from build123d import *

# Parameters (mm, degrees)
SKETCH_1_R               = 2.1
SKETCH_1_W               = 60
SKETCH_1_H               = 60
SKETCH_1_W_2             = 55
SKETCH_1_H_2             = 55
EXTRUDE_1_DEPTH          = 15
CUT_EXTRUDE_1_DEPTH      = 160.024864418
CUT_EXTRUDE_1_DEPTH_BACK = 160.024864418
CUT_EXTRUDE_2_DEPTH      = 184.645620758
CUT_EXTRUDE_2_DEPTH_BACK = 184.645620758


with BuildPart() as part:
    # Эскиз1 → Бобышка-Вытянуть1 (new body)
    # profile 1 of 13: a face of its own
    with BuildSketch(Plane(origin=(0, 45.645974268, 0), x_dir=(-1, 0, 0), z_dir=(0, -1, 0))):
        Polygon((-109.808980694, -130.773129836), (-128.058980694, -130.773129836), (-128.058980694, -48.273129836), (-109.808980694, -48.273129836), (-109.808980694, -53.898129836), (-124.808980694, -53.898129836), (-124.808980694, -125.148129836), (-109.808980694, -125.148129836), align=None)
    # profile 2 of 13: a face of its own
    with BuildSketch(Plane(origin=(0, 45.645974268, 0), x_dir=(-1, 0, 0), z_dir=(0, -1, 0))):
        Polygon((-109.808980694, -130.773129836), (-99.808980694, -130.773129836), (-99.808980694, -124.523129836), (-99.808980694, -119.523129836), (-99.808980694, -95.523129836), (-99.808980694, -83.523129836), (-99.808980694, -59.523129836), (-99.808980694, -54.523129836), (-99.808980694, -48.273129836), (-109.808980694, -48.273129836), (-109.808980694, -53.898129836), (-109.808980694, -125.148129836), align=None)
        with Locations(Location((-104.808980694, -119.523129836, 0), (0, 0, 90))):
            Circle(SKETCH_1_R, mode=Mode.SUBTRACT)
        with Locations(Location((-104.808980694, -59.523129836, 0), (0, 0, 90))):
            Circle(SKETCH_1_R, mode=Mode.SUBTRACT)
    # profile 3 of 13: a face of its own
    with BuildSketch(Plane(origin=(0, 45.645974268, 0), x_dir=(-1, 0, 0), z_dir=(0, -1, 0))):
        with Locations((-64.808980694, -89.523129836)):
            Rectangle(SKETCH_1_W, SKETCH_1_H)
        with Locations((-64.5, -89.5)):
            Rectangle(SKETCH_1_W_2, SKETCH_1_H_2, mode=Mode.SUBTRACT)
    # profile 4 of 13: a face of its own
    with BuildSketch(Plane(origin=(0, 45.645974268, 0), x_dir=(-1, 0, 0), z_dir=(0, -1, 0))):
        Polygon((-64.808980694, -124.523129836), (-55, -124.523129836), (-55, -119.523129836), (-75, -119.523129836), (-75, -124.523129836), align=None)
    # profile 5 of 13: a face of its own
    with BuildSketch(Plane(origin=(0, 45.645974268, 0), x_dir=(-1, 0, 0), z_dir=(0, -1, 0))):
        Polygon((-99.808980694, -130.773129836), (-99.808980694, -124.523129836), (-64.808980694, -124.523129836), (-29.808980694, -124.523129836), (-29.808980694, -130.773129836), align=None)
    # profile 6 of 13: a face of its own
    with BuildSketch(Plane(origin=(0, 45.645974268, 0), x_dir=(-1, 0, 0), z_dir=(0, -1, 0))):
        Polygon((-99.808980694, -54.523129836), (-99.808980694, -48.273129836), (-29.808980694, -48.273129836), (-29.808980694, -54.523129836), (-64.808980694, -54.523129836), align=None)
    # profile 7 of 13: a face of its own
    with BuildSketch(Plane(origin=(0, 45.645974268, 0), x_dir=(-1, 0, 0), z_dir=(0, -1, 0))):
        Polygon((-29.808980694, -130.773129836), (-29.808980694, -124.523129836), (-29.808980694, -54.523129836), (-29.808980694, -48.273129836), (-19.808980694, -48.273129836), (-19.808980694, -53.898129836), (-19.808980694, -125.148129836), (-19.808980694, -130.773129836), align=None)
        with Locations(Location((-24.808980694, -119.523129836, 0), (0, 0, 90))):
            Circle(SKETCH_1_R, mode=Mode.SUBTRACT)
        with Locations(Location((-24.808980694, -59.523129836, 0), (0, 0, 90))):
            Circle(SKETCH_1_R, mode=Mode.SUBTRACT)
    # profile 8 of 13: a face of its own
    with BuildSketch(Plane(origin=(0, 45.645974268, 0), x_dir=(-1, 0, 0), z_dir=(0, -1, 0))):
        Polygon((-4.808980694, -125.148129836), (-4.808980694, -53.898129836), (-19.808980694, -53.898129836), (-19.808980694, -48.273129836), (-1.558980694, -48.273129836), (-1.558980694, -130.773129836), (-19.808980694, -130.773129836), (-19.808980694, -125.148129836), align=None)
    # profile 9 of 13: a face of its own
    with BuildSketch(Plane(origin=(0, 45.645974268, 0), x_dir=(-1, 0, 0), z_dir=(0, -1, 0))):
        Polygon((-99.808980694, -119.523129836), (-99.808980694, -124.523129836), (-94.808980694, -124.523129836), (-89.808980694, -119.523129836), (-94.808980694, -119.523129836), (-94.808980694, -114.523129836), align=None)
    # profile 10 of 13: a face of its own
    with BuildSketch(Plane(origin=(0, 45.645974268, 0), x_dir=(-1, 0, 0), z_dir=(0, -1, 0))):
        Polygon((-34.808980694, -124.523129836), (-29.808980694, -124.523129836), (-29.808980694, -119.523129836), (-34.808980694, -114.523129836), (-34.808980694, -119.523129836), (-39.808980694, -119.523129836), align=None)
    # profile 11 of 13: a face of its own
    with BuildSketch(Plane(origin=(0, 45.645974268, 0), x_dir=(-1, 0, 0), z_dir=(0, -1, 0))):
        Polygon((-34.808980694, -64.523129836), (-29.808980694, -59.523129836), (-29.808980694, -54.523129836), (-34.808980694, -54.523129836), (-39.808980694, -59.523129836), (-34.808980694, -59.523129836), align=None)
    # profile 12 of 13: a face of its own
    with BuildSketch(Plane(origin=(0, 45.645974268, 0), x_dir=(-1, 0, 0), z_dir=(0, -1, 0))):
        Polygon((-99.808980694, -54.523129836), (-99.808980694, -59.523129836), (-94.808980694, -64.523129836), (-94.808980694, -59.523129836), (-89.808980694, -59.523129836), (-94.808980694, -54.523129836), align=None)
    # profile 13 of 13: a face of its own
    with BuildSketch(Plane(origin=(0, 45.645974268, 0), x_dir=(-1, 0, 0), z_dir=(0, -1, 0))):
        Polygon((-55, -59.523129836), (-55, -54.523129836), (-64.808980694, -54.523129836), (-75, -54.523129836), (-75, -59.523129836), align=None)
    extrude(amount=EXTRUDE_1_DEPTH)

    # Эскиз2 → Вырез-Вытянуть1 (cut, two sides: drawn at the far end of the back side and taken through both)
    with BuildSketch(Plane.XY.offset(130.773129836).offset(-CUT_EXTRUDE_1_DEPTH_BACK)):
        Polygon((64.808980694, 44), (72, 44), (72, 37), (58, 37), (58, 44), align=None)
    extrude(amount=CUT_EXTRUDE_1_DEPTH + CUT_EXTRUDE_1_DEPTH_BACK, mode=Mode.SUBTRACT)

    # Эскиз3 → Вырез-Вытянуть2 (cut, two sides: drawn at the far end of the back side and taken through both)
    with BuildSketch(Plane(origin=(0, 45.645974268, 0), x_dir=(1, 0, 0), z_dir=(0, 1, 0)).offset(-CUT_EXTRUDE_2_DEPTH_BACK)):
        Polygon((103.808980694, -70.898129836), (103.808980694, -109.148129836), (109.808980694, -115.148129836), (109.808980694, -63.898129836), align=None)
        Polygon((25.808980694, -70.898129836), (25.808980694, -109.148129836), (19.808980694, -115.148129836), (19.808980694, -63.898129836), align=None)
    extrude(amount=CUT_EXTRUDE_2_DEPTH + CUT_EXTRUDE_2_DEPTH_BACK, mode=Mode.SUBTRACT)


solid = part.part
Geometry: final body of the model. Coordinates: model frame, mm. A direction names the side the tool comes from. Round coordinates to 2 decimals unless told otherwise and drop trailing zeros. Order: outer loops, then holes, each group sorted by start corner. A loop starts at its lowest first (then second) coordinate and runs counter-clockwise, first axis right, second up.
Q1. Section B-B, the plane z = 77. Output: boundary loops of the cut face in (x, y), and give its area (4 significant figures).
Result sheet:
outline: (1.56, 30.65) - (4.81, 30.65) - (4.81, 45.65) - (1.56, 45.65) - close; (25.81, 30.65) - (29.81, 30.65) - (29.81, 45.65) - (25.81, 45.65) - close; (34.81, 30.65) - (37, 30.65) - (37, 45.65) - (34.81, 45.65) - close; (92, 30.65) - (94.81, 30.65) - (94.81, 45.65) - (92, 45.65) - close; (99.81, 30.65) - (103.81, 30.65) - (103.81, 45.65) - (99.81, 45.65) - close; (124.81, 30.65) - (128.06, 30.65) - (128.06, 45.65) - (124.81, 45.65) - close
area: 292.5 mm2
Q2. Material intervals for probe 1 along X at (y, z) = (34.5, 82); probe 2 along Z at (x, y) = (49.5, 39.75); probe 3 along Z at (x, y) = (57, 38.75), sorted ascending.
Result sheet:
probe 1: x = 1.56 to 4.81, 25.81 to 29.81, 34.81 to 37, 92 to 94.81, 99.81 to 103.81, 124.81 to 128.06
probe 2: z = 48.27 to 54.52, 59.52 to 62, 117 to 119.52, 124.52 to 130.77
probe 3: z = 48.27 to 62, 117 to 130.77
Q3. Access query for faces 1 (the face through (65, 37, 124)), 2 (the face through (1.559, 38, 89)), 3 (the face through (109.809, 38, 120)). Directions: +Z, -Z, +X, -X, +Y, -Y. A direction counts if a zero-diameter tool reaches every point of the face in a straight line with its end or side. Return the directions, or none.
Result sheet:
face 1: +Z, -Z
face 2: +Z, -Z, -X, +Y, -Y
face 3: +Y, -Y
Q4. Mould query, pull axis Z, two halves, no side actions, for faces 4 (the face through (97.274, 38.251, 116.988)), 5 (the face through (63.9, 36.6, 130.773)), 6 (the face through (65.7, 36.6, 48.273)), 7 (the face through (128.059, 38, 90)). Classes: released by +Z, released by -Z, zero draft, split by the parting line, or undercut.
Result sheet:
face 4: undercut
face 5: released by +Z
face 6: released by -Z
face 7: zero draft
Q5. Section D-D, the plane x = 41.5. Output: boundary loops of the cut face in (y, z).
Result sheet:
outline: (30.65, 48.27) - (45.65, 48.27) - (45.65, 54.52) - (30.65, 54.52) - close; (30.65, 59.52) - (45.65, 59.52) - (45.65, 62) - (30.65, 62) - close; (30.65, 117) - (45.65, 117) - (45.65, 119.52) - (30.65, 119.52) - close; (30.65, 124.52) - (45.65, 124.52) - (45.65, 130.77) - (30.65, 130.77) - close
Q6. Section C-C, the plane x = 14. Output: boundary loops of the cut face in (y, z), and give its area (3 significant figures).
Result sheet:
outline: (30.65, 48.27) - (45.65, 48.27) - (45.65, 53.9) - (30.65, 53.9) - close; (30.65, 125.15) - (45.65, 125.15) - (45.65, 130.77) - (30.65, 130.77) - close
area: 169 mm2
Q7. Section A-A, the plane x = 70.5. Output: boundary loops of the cut face in (y, z), and give its area (3 significant figures).
Result sheet:
outline: (30.65, 48.27) - (37, 48.27) - (37, 62) - (30.65, 62) - close; (30.65, 117) - (37, 117) - (37, 130.77) - (30.65, 130.77) - close; (44, 48.27) - (45.65, 48.27) - (45.65, 62) - (44, 62) - close; (44, 117) - (45.65, 117) - (45.65, 130.77) - (44, 130.77) - close
area: 220 mm2
